Read the model definition and answer for the solid it produces. Units are mm, in the model's axes. A direction names the side the tool comes from. Round coordinates to 2 decimals unless told otherwise and drop trailing zeros. Write each loop counter-clockwise with the first axis right and the second up, starting at its lowest first coordinate (ties: lowest second). Pieces come first, ordered by that corner, then holes. Notation, with made-up numbers: M -7,-28 L 46,-28 A23 ccw 46,-20 Z; hole C 62,-23.5 d5. An arc over 180 degrees is marked long. Use one line per item in the form item = value. Start each with the question number.
Autodesk Inventor part; units mm, degrees
ref_plane "YZ Plane" through (0, 0, 0) normal (1, 0, 0) x (0, 1, 0)
ref_plane "XZ Plane" through (0, 0, 0) normal (0, 1, 0) x (-1, 0, 0)
ref_plane "XY Plane" through (0, 0, 0) normal (0, 0, 1) x (1, 0, 0)
sketch "Sketch1" plane through (0, 0, 0) normal (0, 0, 1) x (1, 0, 0)
  circle A0 centre (0, 0) radius 19.05
  dimension "d0" = 38.1
extrude "Extrusion1" add sketch "Sketch1" along normal blind 2.54
sketch "Sketch2" plane through (0, 0, 2.54) normal (0, 0, 1) x (1, 0, 0)
  circle A0 centre (0, 0) radius 19.05
  circle A1 centre (0, 0) radius 4.7371
  dimension "d3" = 9.4742
extrude "Extrusion2" add sketch "Sketch2" along normal blind 8.509 contours A1
sketch "Sketch3" plane through (0, 0, 11.049) normal (0, 0, 1) x (1, 0, 0)
  circle A0 centre (0, 0) radius 4.7371
  circle A1 centre (0, 0) radius 1.5177
  dimension "d6" = 3.0353
extrude "Extrusion3" cut sketch "Sketch3" against normal through all contours A1
sketch "Sketch4" plane through (0, 0, 2.54) normal (0, 0, 1) x (1, 0, 0)
  circle A0 centre (0, 0) radius 4.7371
  circle A1 centre (0, 0) radius 19.05
  line L0 (-12.1517, 0.9906) -> (-9.8563, 0.9906)
  line L1 (-0.9906, 12.1517) -> (-0.9906, 9.8563)
  arc A2 (-0.9906, 12.1517) -> (-12.1517, 0.9906) centre (0, 0) ccw
  arc A3 (-0.9906, 9.8563) -> (-9.8563, 0.9906) centre (0, 0) ccw
  dimension "d9" = 0.9906
  dimension "d10" = 0.9906
  dimension "d11" = 9.906
  dimension "d12" = 12.192
extrude "Extrusion4" add sketch "Sketch4" along normal blind 5.08 contours A2 L1 A3 L0
pattern_circular "Circular Pattern1" count 2 over 360 about axis through (0, 0, 0) along (0, 0, 1) of "Extrusion4"
fillet "Fillet1" radius 1.27 1 edges at (-19.05, 0, 0)
equation "\"d10\" = d9"
properties part number "Kornylak Wheel Hub - Out Side"
Q1. Straight lines are drawn through the part: line 1 (Y direction, x = 0, z = 6); line 2 (Y direction, x = 0, z = 2.5); line 3 (Z direction, x = -5.5, y = -15.5). For each, find the intervals that lie inside material, in ascending order. Write a range as [from, to].
Q2. Each of these flat-tipped pins is pushed along its axis until it touches: pin 1 Ø0.7 at (x, z) = (11.5, 4.5) entering from +Y; pin 2 Ø1 at (y, z) = (-7, 8) entering from -X; pin 3 Ø0.7 at (y, z) = (11, 4) entering from +X. Where does it stop, or does it pass through?
Q3. For a pull along X with two mould halves and no side action, classify faces 6 (the face through (-15.12, 11.59, 1.9)), 7 (the face through (0, -2, 11.049)), 8 (the face through (7.07, -6.94, 5.04)) as +X half, -X half, draft (parallel to the pull), parting line (faces both ways), or undercut.
Q4. A tool of negligible diameter and unlimited length cuts with its end or side. For faces 1 (the face through (-7.07, 6.94, 5.04)), 2 (the face through (11, -0.991, 5)), 3 (the face through (0.991, -11, 5)), 4 (the face through (8.706, -8.536, 5.044)), 5 (the face through (-7.4, 7, 7.62)), from which of +Z, -Z, +X, -X, +Y, -Y can it reach the whole face along a straight path? Write none if from no direction.
Q5. Find section D-D on z = 8.5. Write down the section's boundary in (x, y), and give its area (3 significant figures).
Q6. Find section B-B on y = 0. Write down the section's boundary in (x, z).
Q7. Find section A-A on z = 4.75. Write down the section's boundary in (x, y), and give its area (3 significant figures).
Response:
q1.line_1 = [-4.74, -1.52], [1.52, 4.74]
q1.line_2 = [-19.05, -1.52], [1.52, 19.05]
q1.line_3 = [0, 2.54]
q2.pin_1 = -0.99
q2.pin_2 = 6.67
q2.pin_3 = -0.99
q3.face_6 = parting line
q3.face_7 = draft
q3.face_8 = undercut
q4.face_1 = +Z
q4.face_2 = +Z, +X, +Y
q4.face_3 = +Z, -X, -Y
q4.face_4 = +Z, +X, -Y
q4.face_5 = +Z, -X, +Y
q5.outline = C 0,0 d9.47; hole C 0,0 d3.04
q5.area = 63.3 mm²
q6.outline = M -19.05,1.27 A1.27 ccw -17.78,0 L -1.52,0 L -1.52,11.05 L -4.74,11.05 L -4.74,2.54 L -19.05,2.54 Z; M 1.52,0 L 17.78,0 A1.27 ccw 19.05,1.27 L 19.05,2.54 L 4.74,2.54 L 4.74,11.05 L 1.52,11.05 Z
q7.outline = M -12.15,0.99 L -9.86,0.99 A9.91 cw -0.99,9.86 L -0.99,12.15 A12.19 ccw Z; C 0,0 d9.47; M 0.99,-12.15 A12.19 ccw 12.15,-0.99 L 9.86,-0.99 A9.91 cw 0.99,-9.86 Z; hole C 0,0 d3.04
q7.area = 134 mm²
